Design review of the part built by this model. Coordinates are the model's own, in mm. A direction names the side the tool comes from. Coordinates: 2 decimals unless noted, no trailing zeros. Order: outer loops, then holes, each group sorted by start corner. A loop starts at its lowest first (then second) coordinate and runs counter-clockwise, first axis right, second up. Notation, with made-up numbers: (-30.75, 79) -> (3.25, 79) arc R33 cw to (3.25, 109) -> close; hole circle Ø3 at (-35.5, 37.25). An arc over 180 degrees is marked (long way). Write item = value, one per line.
```python
from build123d import *

# Parameters (mm, degrees)
SKETCH7_R                       = 2.4892
CUT_EXTRUDE1_DEPTH              = 89.9
F_21_0_159_DIAMETER_HOLE1_D     = 4.0386
F_21_0_159_DIAMETER_HOLE1_DEPTH = 17.78
F_21_0_159_DIAMETER_HOLE1_TIP   = 1.213317848
SKETCH15_R                      = 2.413
CUT_EXTRUDE2_DEPTH              = 4.826


with BuildPart() as part:
    # Sketch1 → Revolve1 (revolve)
    with BuildSketch(Plane.XY):
        Polygon((-88.9, 53.848), (-88.9, 44.45), (0, 44.45), (0, 63.5), (-12.7, 63.5), (-12.7, 53.848), align=None)
    revolve(axis=Axis((-87.283636364, 0, 0), (1, 0, 0)))

    # Sketch7 → Cut-Extrude1 (cut, through all)
    with BuildSketch(Plane(origin=(0, 0, 0), x_dir=(0, 0, -1), z_dir=(1, 0, 0))):
        with Locations((-16.571472984, 56.020377392)):
            Circle(SKETCH7_R)
        with Locations((13.658872113, 56.800806443)):
            Circle(SKETCH7_R)
        with Locations((40.229333459, 42.361505278)):
            Circle(SKETCH7_R)
        with Locations((56.020377392, 16.571472984)):
            Circle(SKETCH7_R)
        with Locations((56.800806443, -13.658872113)):
            Circle(SKETCH7_R)
        with Locations((42.361505278, -40.229333459)):
            Circle(SKETCH7_R)
        with Locations((16.571472984, -56.020377392)):
            Circle(SKETCH7_R)
        with Locations((-13.658872113, -56.800806443)):
            Circle(SKETCH7_R)
        with Locations((-40.229333459, -42.361505278)):
            Circle(SKETCH7_R)
        with Locations((-56.020377392, -16.571472984)):
            Circle(SKETCH7_R)
        with Locations((-56.800806443, 13.658872113)):
            Circle(SKETCH7_R)
        with Locations((-42.361505278, 40.229333459)):
            Circle(SKETCH7_R)
    extrude(amount=-CUT_EXTRUDE1_DEPTH, mode=Mode.SUBTRACT)

    # #21 (0.159) Diameter Hole1
    with Locations(Plane.ZY.offset(88.9)):
        with Locations((-33.845113149, 35.638918571), (1.268411978, 49.132630014), (35.638918571, 33.845113149), (49.132630014, -1.268411978), (33.845113149, -35.638918571), (-1.268411978, -49.132630014), (-35.638918571, -33.845113149), (-49.132630014, 1.268411978)):
            Hole(F_21_0_159_DIAMETER_HOLE1_D / 2, depth=F_21_0_159_DIAMETER_HOLE1_DEPTH)
            with Locations((0, 0, -(F_21_0_159_DIAMETER_HOLE1_DEPTH + F_21_0_159_DIAMETER_HOLE1_TIP / 2))):  # 118° drill point
                Cone(0, F_21_0_159_DIAMETER_HOLE1_D / 2, F_21_0_159_DIAMETER_HOLE1_TIP, mode=Mode.SUBTRACT)

    # Sketch15 → Cut-Extrude2 (cut)
    with BuildSketch(Plane(origin=(0, 0, 0), x_dir=(0, 0, -1), z_dir=(1, 0, 0))):
        with Locations((-1.507673152, 58.400542135)):
            Circle(SKETCH15_R)
        with Locations((1.507673152, -58.400542135)):
            Circle(SKETCH15_R)
    extrude(amount=-CUT_EXTRUDE2_DEPTH, mode=Mode.SUBTRACT)


solid = part.part
```
(1) The part is to be moulded in two halves that separate along Y. For faces 4 (the flat face through (-12.7, 19, -51)), 5 (the cylindrical face through (-6.261, 42.471, -37.743)), say which applies: released by +Y, released by -Y, zero draft, split by the parting line, or undercut.
Report:
face_4 = zero draft
face_5 = undercut
(2) We need section B-B (y = -23.5). Write out the cut boundary in (x, z).
Report:
outline = (-88.9, -48.45) -> (-12.7, -48.45) -> (-12.7, -58.99) -> (0, -58.99) -> (0, -37.73) -> (-88.9, -37.73) -> close; (-88.9, 37.73) -> (0, 37.73) -> (0, 58.99) -> (-12.7, 58.99) -> (-12.7, 48.45) -> (-88.9, 48.45) -> close
(3) Insertion check: pin 1 (4 mm diameter, centred on x = -40.5, y = -17, fed in from -Z); pin 2 (2.5 mm diameter, centred on y = 35.64, z = -33.85, fed in from -X); pin 3 (3 mm diameter, centred on y = 13.66, z = 56.8, fed in from -X); pin 4 (6 mm diameter, centred on x = -9, z = -18, fed in from +Y). Each pin has a flat end and moves straight along its axis. Give the tip position at first contact, or say it passes through.
Report:
pin_1 = -51.72
pin_2 = -70.66
pin_3 = through
pin_4 = 61.7
(4) For faces 1 (the cylindrical face through (-6.261, 58.488, 16.896)), 2 (the cylindrical face through (-2.379, -56.366, -2.805)), 3 (the cylindrical face through (-79.886, 47.161, 1.706)), list the 3-axis set-ups (+Z, -Z, +X, -X, +Y, -Y) from which the entire face can be reached by the end or side of a thin tool; tool diameter is ignored.
Report:
face_1 = +X, -X
face_2 = +X
face_3 = -X
(5) We need section A-A (x = -75). Give the number of separate pieces and of enclosed holes in the cut face, and give its area (3 significant figures).
Report:
separate_pieces = 1
enclosed_holes = 9
area = 2,800 mm²
(6) We need section C-C (x = -62.5). Write out the cut boundary in (y, z).
Report:
outline = circle Ø107.7 at (0, 0); hole circle Ø88.9 at (0, 0)
(7) For L1, parallel to Y at x = -27, z = -1; L2, parallel to Y at x = -82, z = 35.5; L3, parallel to Z at x = -85, y = -34, list the stretches that pass through material, from the lowest coordinate up.
Report:
L1 = -53.84 to -44.44, 44.44 to 53.84
L2 = -40.49 to -36.8, -34.48 to -26.75, 26.75 to 31.83, 35.86 to 40.49
L3 = -41.76 to -37.65, -33.63 to -28.63, 28.63 to 32.67, 35.02 to 41.76
